Here's how the part is built. I have some questions about the finished solid (model axes, mm). Coordinates: 2 decimals unless noted, no trailing zeros. Write each loop counter-clockwise with the first axis right and the second up, starting at its lowest first coordinate (ties: lowest second). Pieces come first, ordered by that corner, then holes. Notation, with made-up numbers: M 23.5,-21.5 L 65.5,-21.5 A9 ccw 65.5,-13.5 Z; hole C 8,76.25 d5. An arc over 180 degrees is marked long. Use a Markdown table: item, result.
```python
from build123d import *

# Parameters (mm, degrees)
F0_W     = 611.7065250874
F0_H     = 284.1202020645
F1_DEPTH = 508
F2_W     = 611.7065250874
F2_H     = 384.5913410187
F3_DEPTH = 127
F6_DEPTH = 535.686
F7_DEPTH = 254


with BuildPart() as f1:
    # F0 (on Front) → F1 (new body)
    with BuildSketch(Plane.XZ):
        with Locations((36.3153368235, -2.8254389763)):
            Rectangle(F0_W, F0_H)
    extrude(amount=F1_DEPTH)

    # F2 (on face) → F3 (join)
    with BuildSketch(Plane.XY.offset(139.234662056)):
        with Locations((36.3153368235, -192.2956705093)):
            Rectangle(F2_W, F2_H)
    extrude(amount=F3_DEPTH)

    # F5 (on face) → F6 (join)
    with BuildSketch(Plane(origin=(-269.5379257202, 0, 0), x_dir=(0, -1, 0), z_dir=(-1, 0, 0))):
        Polygon((508, 139.234662056), (384.5913410187, 266.234662056), (384.5913410187, 139.234662056), align=None)
    extrude(amount=-F6_DEPTH)

    # F4 (on face) → F7 (join)
    with BuildSketch(Plane.YZ.offset(342.1685993671)):
        Polygon((-384.5913410187, 139.234662056), (-384.5913410187, 266.234662056), (-508, 139.234662056), align=None)
    extrude(amount=-F7_DEPTH)


solid = f1.part
```
1. Will this pin go through, and if not, where does the flat tip stop? pin 1 Ø5 at (x, y) = (-169.5, -410.5) entering from +Z.
Answers follow:
| item | result |
|---|---|
| pin 1 | stops at z = 242.14 |
2. Suppose I cut it at C-C on y = -454.5. Write out the boundary of the cut face in (x, z).
Answers follow:
| item | result |
|---|---|
| outline | M -269.54,-144.89 L 342.17,-144.89 L 342.17,194.29 L -269.54,194.29 Z |
3. I need wall thicknesses on probe 1 along Y at (x, z) = (-18.5, 199); probe 2 along Y at (x, z) = (254, 198); probe 3 along Z at (x, y) = (65.5, -441). Which ranges of each line are inside material? Lowest first, please.
Answers follow:
| item | result |
|---|---|
| probe 1 | y = -449.92 to 0 |
| probe 2 | y = -450.9 to 0 |
| probe 3 | z = -144.89 to 208.18 |
4. Suppose I cut it at A-A on x = 267. Write out the boundary of the cut face in (y, z), and give its area (3 significant figures).
Answers follow:
| item | result |
|---|---|
| outline | M -508,-144.89 L 0,-144.89 L 0,266.23 L -384.59,266.23 L -508,139.23 Z |
| area | 201,000 mm2 |
5. Suppose I cut it at B-B on z = 150. Write out the boundary of the cut face in (x, y).
Answers follow:
| item | result |
|---|---|
| outline | M -269.54,-497.54 L 342.17,-497.54 L 342.17,0 L -269.54,0 Z |
